from build123d import *

# Parameters (mm, degrees)
MAINBODY_DEPTH      = 10
SCREWCUTOUTS_DEPTH  = 205.863369102
SKETCH2_R           = 4
SKETCH2_R_2         = 1.45
RODCUTOUTS_DEPTH    = 205.863369102
SKETCH4_R           = 1.45
SKETCH4_W           = 9.85
SKETCH4_H           = 9.7
CUT_EXTRUDE3_DEPTH  = 205.863369102
SKETCH5_R           = 1.45
SKETCH5_W           = 4.35
SKETCH5_H           = 9.7
SKETCH5_H_2         = 9.9
ENDSTOPHOLDER_DEPTH = 205.863369102
CUT_EXTRUDE4_DEPTH  = 205.863369102


with BuildPart() as part:
    # Sketch1 → MainBody (new body)
    with BuildSketch(Plane.XY):
        Polygon((0, 0), (-185, 0), (-185, -24), (-195, -24), (-195, -34), (-185, -34), (-185, -48), (-195, -48), (-195, -58), (-185, -58), (-185, -62), (0, -62), align=None)
    mainbody = extrude(amount=MAINBODY_DEPTH)

    # Sketch3 → ScrewCutouts (cut, through all)
    with BuildSketch(Plane.XY.offset(10)):
        with BuildLine():
            Line((-185, -18.55), (-180.5, -18.55))
            Line((-180.5, -18.55), (-180.5, -19.35))
            ThreePointArc((-180.5, -19.35), (-180.353553391, -19.703553391), (-180, -19.85))
            Line((-180, -19.85), (-177.5, -19.85))
            ThreePointArc((-177.5, -19.85), (-177.146446609, -19.703553391), (-177, -19.35))
            Line((-177, -19.35), (-177, -18.55))
            Line((-177, -18.55), (-174, -18.55))
            Line((-174, -18.55), (-174, -15.45))
            Line((-174, -15.45), (-177, -15.45))
            Line((-177, -15.45), (-177, -14.65))
            ThreePointArc((-177, -14.65), (-177.146446609, -14.296446609), (-177.5, -14.15))
            Line((-177.5, -14.15), (-180, -14.15))
            ThreePointArc((-180, -14.15), (-180.353553391, -14.296446609), (-180.5, -14.65))
            Line((-180.5, -14.65), (-180.5, -15.45))
            Line((-180.5, -15.45), (-185, -15.45))
            Line((-185, -15.45), (-185, -18.55))
        make_face()
        with BuildLine():
            Line((-185, -39.45), (-185, -42.55))
            Line((-185, -42.55), (-180.5, -42.55))
            Line((-180.5, -42.55), (-180.5, -43.35))
            ThreePointArc((-180.5, -43.35), (-180.353553391, -43.703553391), (-180, -43.85))
            Line((-180, -43.85), (-177.5, -43.85))
            ThreePointArc((-177.5, -43.85), (-177.146446609, -43.703553391), (-177, -43.35))
            Line((-177, -43.35), (-177, -42.55))
            Line((-177, -42.55), (-174, -42.55))
            Line((-174, -42.55), (-174, -39.45))
            Line((-174, -39.45), (-177, -39.45))
            Line((-177, -39.45), (-177, -38.65))
            ThreePointArc((-177, -38.65), (-177.146446609, -38.296446609), (-177.5, -38.15))
            Line((-177.5, -38.15), (-180, -38.15))
            ThreePointArc((-180, -38.15), (-180.353553391, -38.296446609), (-180.5, -38.65))
            Line((-180.5, -38.65), (-180.5, -39.45))
            Line((-180.5, -39.45), (-185, -39.45))
        make_face()
    screwcutouts = extrude(amount=-SCREWCUTOUTS_DEPTH, mode=Mode.SUBTRACT)

    # Mirror1: MainBody, ScrewCutouts across plane
    add(mainbody.mirror(Plane(origin=(0, 0, 0), x_dir=(0, 0, 1), z_dir=(1, 0, 0))))
    add(screwcutouts.mirror(Plane(origin=(0, 0, 0), x_dir=(0, 0, 1), z_dir=(1, 0, 0))), mode=Mode.SUBTRACT)

    # Sketch2 → RodCutouts (cut, through all)
    with BuildSketch(Plane.XY.offset(10)):
        with Locations((-73, -3.5)):
            Circle(SKETCH2_R)
        with Locations((-83, -4.5)):
            Circle(SKETCH2_R_2)
        with Locations(Location((-63, -4.5, 0), (0, 0, 180))):
            Circle(SKETCH2_R_2)
        with Locations((67, -4.5)):
            Circle(SKETCH2_R_2)
        with Locations(Location((87, -4.5, 0), (0, 0, 180))):
            Circle(SKETCH2_R_2)
        with Locations((77, -3.5)):
            Circle(SKETCH2_R)
    extrude(amount=-RODCUTOUTS_DEPTH, mode=Mode.SUBTRACT)

    # Sketch4 → Cut-Extrude3 (cut, through all)
    with BuildSketch(Plane.XY.offset(10)):
        with Locations((7, -25)):
            Circle(SKETCH4_R)
        with Locations((7, -10)):
            Rectangle(SKETCH4_W, SKETCH4_H)
        with Locations((7, -40)):
            Rectangle(SKETCH4_W, SKETCH4_H)
    extrude(amount=-CUT_EXTRUDE3_DEPTH, mode=Mode.SUBTRACT)

    # Sketch5 → EndstopHolder (cut, through all)
    with BuildSketch(Plane.XY.offset(10)):
        with Locations((-41, -37.75)):
            Circle(SKETCH5_R)
        with Locations((-41, -22.8)):
            Rectangle(SKETCH5_W, SKETCH5_H)
        with Locations((-41, -52.8)):
            Rectangle(SKETCH5_W, SKETCH5_H_2)
        with BuildLine():
            Line((-31.425, 8.994431211), (-31.425, 5))
            ThreePointArc((-31.425, 5), (-34.625, 1.8), (-37.825, 5))
            Line((-37.825, 5), (-37.825, 8.994431211))
            ThreePointArc((-37.825, 8.994431211), (-34.625, 12.194431211), (-31.425, 8.994431211))
        make_face()
    extrude(amount=-ENDSTOPHOLDER_DEPTH, mode=Mode.SUBTRACT)

    # Sketch7 → Cut-Extrude4 (cut, through all)
    with BuildSketch(Plane.XY.offset(10)):
        with BuildLine():
            Line((-98.5, 0), (-98.5, -2))
            ThreePointArc((-98.5, -2), (-102.5, -6), (-106.5, -2))
            Line((-106.5, -2), (-106.5, 0))
            ThreePointArc((-106.5, 0), (-102.5, 4), (-98.5, 0))
        make_face()
        with BuildLine():
            Line((102.5, 0), (102.5, -2))
            ThreePointArc((102.5, -2), (106.5, -6), (110.5, -2))
            Line((110.5, -2), (110.5, 0))
            ThreePointArc((110.5, 0), (106.5, 4), (102.5, 0))
        make_face()
    extrude(amount=-CUT_EXTRUDE4_DEPTH, mode=Mode.SUBTRACT)


solid = part.part
The model under review builds one solid part; all positions refer to its coordinate system, in mm. A direction names the side the tool comes from. Give positions to 0.01 mm unless a question says otherwise; leave off trailing zeros. Write item = value, one per line. Start each with the question number.
(1) For L1, parallel to Y at x = -41, z = 5.75; L2, parallel to X at y = -51.5, z = 2.25 (3 decimals); L3, parallel to X at y = -39.5, z = 8.5 (3 decimals), list the stretches that pass through material, from the lowest coordinate up. Write a range as from..to.
(2) For pin 1 Ø1.5 at (y, z) = (-17, 1.5) entering from -X; pin 2 Ø5 at (y, z) = (-41.5, 4) entering from -X, all flat-tipped, find the tip position at first contact; note any pin that passes through.
(3) Draft analysis for pull direction Y (two halves, no side actions). For faces 5 (the flat face through (-43.175, -23, 5)), 6 (the flat face through (190, -24, 5)), 7 (the flat face through (195, -53, 5)), state which applies: +Y half, -Y half, draft (parallel to the pull), parting line (faces both ways), or undercut.
(4) Take a section at A-A (z = 7.5). State how many separate pieces and enclosed holes the cut face has, plus the area to 3 significant figures.
(5) Tool access review of faces 1 (the flat face through (190, -48, 5)), 2 (the flat face through (190, -58, 5)), 3 (the flat face through (-43.175, -53, 5)), 4 (the flat face through (-190, -48, 5)): name each direction out of +Z, -Z, +X, -X, +Y, -Y from which nothing blocks a thin tool from reaching the whole face with its end or side.
Returned:
q1.L1 = -62..-57.75, -47.85..-39.2, -36.3..-27.65, -17.95..0
q1.L2 = -195..-43.175, -38.825..195
q1.L3 = -174..2.075, 11.925..174
q2.pin_1 = -174
q2.pin_2 = -185
q3.face_5 = undercut
q3.face_6 = +Y half
q3.face_7 = draft
q4.separate_pieces = 1
q4.enclosed_holes = 10
q4.area = 22,700 mm²
q5.face_1 = +Z, -Z, +X
q5.face_2 = +Z, -Z, +X, -Y
q5.face_3 = +Z, -Z
q5.face_4 = +Z, -Z, -X
